The listing builds one solid part. Answer for the finished solid, in the listing's coordinates (mm). Coordinates: 2 decimals unless noted, no trailing zeros. Loops run counter-clockwise (first coordinate to the right, second up) from the corner with the lowest first, then second, coordinate; pieces in that order, holes last. Notation, with made-up numbers: (6, 67.25) - (14, 67.25) arc R19 ccw to (14, 90.25) - close; hole circle Ø10 at (54.25, 68). An arc over 180 degrees is marked (long way). Use one line per item in the form item = value. Start each with the question number.
```python
from build123d import *

# Parameters (mm, degrees)
CROQUIS1_R              = 4
SALIENTE_EXTRUIR1_DEPTH = 5
CORTAR_EXTRUIR2_DEPTH   = 6


with BuildPart() as part:
    # Croquis1 → Saliente-Extruir1 (new body)
    with BuildSketch(Plane(origin=(0, 0, 0), x_dir=(1, 0, 0), z_dir=(0, 1, 0))):
        with BuildLine():
            Line((-303, 250), (303, 250))
            ThreePointArc((303, 250), (315.02081528, 245.02081528), (320, 233))
            Line((320, 233), (320, -233))
            ThreePointArc((320, -233), (315.02081528, -245.02081528), (303, -250))
            Line((303, -250), (-303, -250))
            ThreePointArc((-303, -250), (-315.02081528, -245.02081528), (-320, -233))
            Line((-320, -233), (-320, 233))
            ThreePointArc((-320, 233), (-315.02081528, 245.02081528), (-303, 250))
        make_face()
        with Locations((0, 235)):
            Circle(CROQUIS1_R, mode=Mode.SUBTRACT)
        with Locations((305, 235)):
            Circle(CROQUIS1_R, mode=Mode.SUBTRACT)
        with Locations((-305, 235)):
            Circle(CROQUIS1_R, mode=Mode.SUBTRACT)
        with Locations((0, -235)):
            Circle(CROQUIS1_R, mode=Mode.SUBTRACT)
        with Locations((305, -235)):
            Circle(CROQUIS1_R, mode=Mode.SUBTRACT)
        with Locations((-305, -235)):
            Circle(CROQUIS1_R, mode=Mode.SUBTRACT)
    extrude(amount=SALIENTE_EXTRUIR1_DEPTH)

    # Croquis3 → Cortar-Extruir2 (cut, through all)
    with BuildSketch(Plane.XZ):
        with BuildLine():
            Line((-227, 60), (-320, 60))
            Line((-320, 60), (-320, -60))
            Line((-320, -60), (-227, -60))
            ThreePointArc((-227, -60), (-167, 0), (-227, 60))
        make_face()
    extrude(amount=-CORTAR_EXTRUIR2_DEPTH, mode=Mode.SUBTRACT)


solid = part.part
```
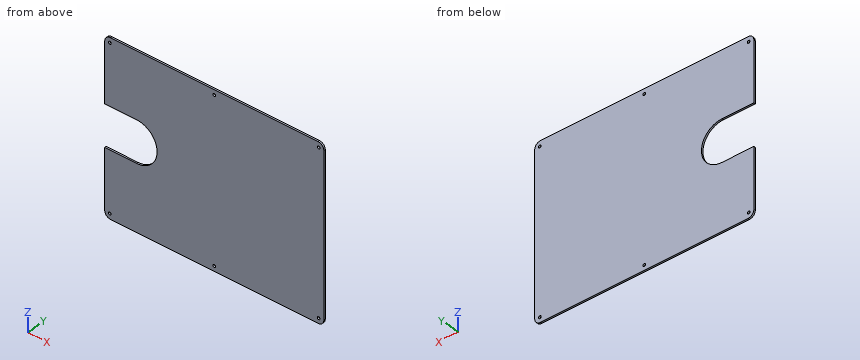
(1) A cutting plane is placed at C-C (z = 0). Determine the outline of the cut face in (x, y), then the cut area to 4 significant figures.
(2) A cutting plane is placed at B-B (x = -201). Determine the outline of the cut face in (y, z).
(3) This flat-tipped pin is pushed along its axis until it touches: pin 1 Ø7 at (x, z) = (-305, 235) entering from -Y. Where does it stop, or does it pass through?
(4) Find the intervals of material crossed by probe 1 along Z at (x, y) = (-305, 1.6); probe 2 along X at (y, z) = (3.2, 235); probe 3 along Z at (x, y) = (0, 1.9), in increasing order. Write a range as from..to.
(5) A cutting plane is placed at A-A (y = 2.2). Determine the outline of the cut face in (x, z), then the cut area to 3 significant figures.
Evaluation:
q1.outline = (-167, 0) - (320, 0) - (320, 5) - (-167, 5) - close
q1.area = 2,435 mm^2
q2.outline = (0, -250) - (5, -250) - (5, -54.07) - (0, -54.07) - close; (0, 54.07) - (5, 54.07) - (5, 250) - (0, 250) - close
q3.pin_1 = through
q4.probe_1 = -249.88..-239, -231..-60, 60..231, 239..249.88
q4.probe_2 = -319.88..-309, -301..-4, 4..301, 309..319.88
q4.probe_3 = -250..-239, -231..231, 239..250
q5.outline = (-320, -233) arc R17 ccw to (-303, -250) - (303, -250) arc R17 ccw to (320, -233) - (320, 233) arc R17 ccw to (303, 250) - (-303, 250) arc R17 ccw to (-320, 233) - (-320, 60) - (-227, 60) arc R60 cw to (-227, -60) - (-320, -60) - close; hole circle Ø8 at (-305, -235); hole circle Ø8 at (-305, 235); hole circle Ø8 at (0, -235); hole circle Ø8 at (0, 235); hole circle Ø8 at (305, -235); hole circle Ø8 at (305, 235)
q5.area = 303,000 mm^2
